Autodesk Inventor part; units mm, degrees
ref_plane "YZ Plane" through (0, 0, 0) normal (1, 0, 0) x (0, 1, 0)
ref_plane "XZ Plane" through (0, 0, 0) normal (0, 1, 0) x (-1, 0, 0)
ref_plane "XY Plane" through (0, 0, 0) normal (0, 0, 1) x (1, 0, 0)
sketch "Sketch1" plane through (0, 0, 0) normal (1, 0, 0) x (0, 1, 0)
  line L0 (-225, -125) -> (225, -125)
  line L1 (225, -125) -> (225, -25)
  line L2 (75, 125) -> (-225, 125)
  line L3 (-225, 125) -> (-225, -125)
  line L4 (-225, -125) -> (225, 125) construction
  line L5 (225, -125) -> (-225, 125) construction
  arc A0 (225, -25) -> (75, 125) centre (75, -25) ccw
  point P0 (0, 0)
  dimension "d0" = 450
  dimension "d1" = 250
  dimension "d2" = 150
extrude "Extrusion1" add sketch "Sketch1" along normal mid plane 390
shell "Shell1" thickness 2 removed faces 1 at (65, -75, -125)
sketch "Sketch2" plane through (195, 225, -125) normal (0, 0, -1) x (-1, 0, 0)
  line L0 (2, -448) -> (2, -2)
  line L1 (2, -2) -> (388, -2)
  line L2 (388, -2) -> (388, -448)
  line L3 (388, -2) -> (388, -448)
  line L4 (2, -448) -> (2, -2)
  line L5 (2, -2) -> (388, -2)
  line L6 (442, -450) -> (442, 44)
  line L7 (442, 44) -> (-52, 44)
  line L8 (-52, 44) -> (-52, -450)
  line L9 (0, -450) -> (390, -450)
  line L10 (2, -448) -> (2, -450)
  line L11 (388, -448) -> (388, -450)
  line L12 (-52, -450) -> (2, -450)
  line L13 (388, -450) -> (442, -450)
  point P0 (195, -225)
  point P1 (195, -450)
  dimension "d6" = 494
  dimension "d7" = 494
sketch "Sketch3" plane through (-193, -223, -125) normal (0, 1, 0) x (1, 0, 0)
  line L0 (0, 0) -> (386, 0)
  line L1 (0, 0) -> (0, -248)
  line L2 (0, -248) -> (386, -248)
  line L3 (386, -248) -> (386, 0)
  point P0 (193, -125)
extrude "Extrusion2" cut sketch "Sketch3" against normal blind 2
extrude "Extrusion3" add sketch "Sketch2" along normal blind 2 contours L10 L9 L12 L8 L7 L6 L13 L11 L2 L1 L0
hole "Hole1" at (-222, 244, -127) direction (0, 0, 1) diameter 6 end through all
pattern_linear "Rectangular Pattern1" count 3 spacing 222 along (1, 0, 0) count 3 spacing 222 along (0, -1, 0) of "Hole1"
properties part number "SidePanelCover-Curved"
Part model, mm, in its own coordinate system. A direction names the side the tool comes from. Round coordinates to 2 decimals unless told otherwise and drop trailing zeros. Loops run counter-clockwise (first coordinate to the right, second up) from the corner with the lowest first, then second, coordinate; pieces in that order, holes last. Notation, with made-up numbers: (18, 23) -> (41, 23) arc R20 cw to (41, 35) -> close; hole circle Ø4 at (41, 1). An arc over 180 degrees is marked (long way). Use one line per item in the form item = value. Start each with the question number.
Item 1: Band-saw the part on C-C (y = -126.5). List the corners of the cut face in (x, z), plus the area to 3 significant figures.
Item 2: Tool access for faces 5 (the flat face through (-195, -3, 2)), 6 (the flat face through (-3, -73, 123)), 7 (the flat face through (-3, -73, 125)): list every direction of +Z, -Z, +X, -X, +Y, -Y with a clear straight run to the whole face (end or side of a thin tool).
Item 3: Band-saw the part on B-B (x = 99). List the corners of the cut face in (y, z).
Item 4: Two-plate mould, pull along X, no slides. Class faces 1 (the flat face through (3, 223, -75)), 2 (the flat face through (-3, 225, -76)), 3 (the flat face through (195, -3, 2)), 4 (the cylindrical face through (-2.7, 178.49, 80.8)): released by +X, released by -X, zero draft, split by the parting line, or undercut.
Item 5: Band-saw the part on D-D (y = 196). List the corners of the cut face in (x, z).
Item 6: Drill centre lines: line 1 along Y through (x, z) = (-222, -126.05); line 2 along X through (y, z) = (22, -126.55); line 3 along X through (y, z) = (244, -125.8). Where is each one in solid material? Low to high.
Item 7: Band-saw the part on A-A (z = -66). List the corners of the cut face in (x, y), plus the area to 3 significant figures.
Item 8: Drop flat-ended pins along their axis: pin 1 Ø8 at (x, y) = (-222, 22) entering from +Z; pin 2 Ø3 at (x, z) = (179.5, -51.5) entering from +Y; pin 3 Ø5.5 at (x, y) = (222, 244) entering from +Z; pin 4 Ø3 at (y, z) = (-147, 68) entering from +X. Give the stop position or say it passes through.
Data:
q1.outline = (-247, -127) -> (-193, -127) -> (-193, 123) -> (193, 123) -> (193, -127) -> (247, -127) -> (247, -125) -> (195, -125) -> (195, 125) -> (-195, 125) -> (-195, -125) -> (-247, -125) -> close
q1.area = 1,990 mm^2
q2.face_5 = +Z, -X, +Y, -Y
q2.face_6 = -Z, -Y
q2.face_7 = +Z, +X, -X, +Y, -Y
q3.outline = (-225, 123) -> (75, 123) arc R148 cw to (223, -25) -> (223, -127) -> (269, -127) -> (269, -125) -> (225, -125) -> (225, -25) arc R150 ccw to (75, 125) -> (-225, 125) -> close
q4.face_1 = undercut
q4.face_2 = zero draft
q4.face_3 = released by +X
q4.face_4 = undercut
q5.outline = (-247, -127) -> (-193, -127) -> (-193, 60.22) -> (193, 60.22) -> (193, -127) -> (247, -127) -> (247, -125) -> (195, -125) -> (195, 63.65) -> (-195, 63.65) -> (-195, -125) -> (-247, -125) -> close
q6.line_1 = -225 to -203, -197 to 19, 25 to 241, 247 to 269
q6.line_2 = -247 to -225, -219 to -193, 193 to 219, 225 to 247
q6.line_3 = -247 to -225, -219 to -3, 3 to 219, 225 to 247
q7.outline = (-195, -225) -> (-193, -225) -> (-193, 223) -> (193, 223) -> (193, -225) -> (195, -225) -> (195, 225) -> (-195, 225) -> close
q7.area = 2,570 mm^2
q8.pin_1 = -125
q8.pin_2 = 225
q8.pin_3 = through
q8.pin_4 = 195
